Geometry: final body of the model. Coordinates: model frame, mm. A direction names the side the tool comes from. Round coordinates to 2 decimals unless told otherwise and drop trailing zeros. Write each loop counter-clockwise with the first axis right and the second up, starting at its lowest first coordinate (ties: lowest second). Pieces come first, ordered by that corner, then holes. Notation, with made-up numbers: (15.5, 24.25) - (46.5, 24.25) arc R15 ccw to (46.5, 29.25) - close; hole circle Ø6 at (-25.75, 54.25). An arc over 180 degrees is marked (long way). Write each question's results on one line, items separated by ' | '.
from build123d import *

# Parameters (mm, degrees)
SKETCH_2_R               = 15
EXTRUDE_1_DEPTH          = 13
SKETCH_8_R               = 2
CUT_EXTRUDE_10_DEPTH     = 12.5
EXTRUDE_START            = 0.5
SKETCH_10_R              = 15
EXTRUDE_4_DEPTH          = 0.5
SKETCH_11_R              = 12
EXTRUDE_5_DEPTH          = 0.5
SKETCH_12_R              = 5
CUT_EXTRUDE_12_DEPTH     = 26.416530054
FILLET_START             = -0.3000001
FILLET_2_DEPTH           = 13.1000002
FILLET_2_2_ANGLE         = 17.614798
PATTERN_CIRCULAR_1_COUNT = 20


with BuildPart() as part:
    # 草图2 → 凸台-拉伸1 (new body)
    with BuildSketch(Plane(origin=(0, 0, 0), x_dir=(1, 0, 0), z_dir=(0, 1, 0))):
        with Locations(Location((0, 0, 0), (0, 0, 90))):
            Circle(SKETCH_2_R)
    extrude(amount=EXTRUDE_1_DEPTH)

    # 草图8 → 切除-拉伸10 (cut)
    with BuildSketch(Plane.XZ):
        with Locations((0, 15)):
            Circle(SKETCH_8_R)
    cut_extrude_10 = extrude(amount=-CUT_EXTRUDE_10_DEPTH, mode=Mode.SUBTRACT)

    # 草图10 → 凸台-拉伸4 (add)
    with BuildSketch(Plane.XZ.offset(EXTRUDE_START)):
        with Locations(Location((0, 0, 0), (0, 0, 270))):
            Circle(SKETCH_10_R)
    extrude(amount=-EXTRUDE_4_DEPTH)

    # 草图11 → 凸台-拉伸5 (add)
    with BuildSketch(Plane.XZ.offset(0.5)):
        with Locations(Location((0, 0, 0), (0, 0, 270))):
            Circle(SKETCH_11_R)
    extrude(amount=EXTRUDE_5_DEPTH)

    # 草图12 → 切除-拉伸12 (cut, through all)
    with BuildSketch(Plane.XZ.offset(1)):
        with Locations(Location((0, 0, 0), (0, 0, 270))):
            Circle(SKETCH_12_R)
    extrude(amount=-CUT_EXTRUDE_12_DEPTH, mode=Mode.SUBTRACT)

    # 圆角2: read off the stored shape, not the designer's step
    # 圆角2 outline → 圆角2 (cut)
    with BuildSketch(Plane(origin=(0, 0, 0), x_dir=(1, 0, 0), z_dir=(0, 1, 0)).offset(FILLET_START)):
        with BuildLine():
            ThreePointArc((2.296701806, -14.823129252), (2.080163818, -14.773434354), (1.957189365, -14.588405797))
            ThreePointArc((1.957189365, -14.588405797), (0, -13), (-1.957189365, -14.588405797))
            ThreePointArc((-1.957189365, -14.588405797), (-2.080163818, -14.773434354), (-2.296701806, -14.823129252))
            ThreePointArc((-2.296701806, -14.823129252), (0, -15), (2.296701806, -14.823129252))
        make_face()
    extrude(amount=FILLET_2_DEPTH, mode=Mode.SUBTRACT)

    # Fillet 2 2 outline → Fillet 2 2 (revolve)
    with BuildSketch(Plane(origin=(0, 0, 0), x_dir=(-0.1531134537578896, 0, 0.9882086167800453), z_dir=(-0.9882086167800453, 0, -0.1531134537578896))):
        with BuildLine():
            Line((13, 12.8000001), (13, 12.5))
            Line((13, 12.5), (14.7, 12.5))
            ThreePointArc((14.7, 12.5), (14.912132034, 12.587867966), (15, 12.8))
            Line((15, 12.8), (13, 12.8000001))
        make_face()
        with BuildLine():
            Line((14.7, 0), (13, 0))
            Line((13, 0), (13, -0.3000001))
            Line((13, -0.3000001), (15, -0.3))
            ThreePointArc((15, -0.3), (14.912132034, -0.087867966), (14.7, 0))
        make_face()
    revolve(axis=Axis((0, 0, 0), (0, 1, 0)), revolution_arc=FILLET_2_2_ANGLE)

    # 阵列(圆周)1: 切除-拉伸10 ×20 about axis
    pattern_circular_1_axis = Axis((0, 0, 0), (0, 1, 0))
    for i in range(1, PATTERN_CIRCULAR_1_COUNT):
        add(cut_extrude_10.rotate(pattern_circular_1_axis, i * 360 / PATTERN_CIRCULAR_1_COUNT), mode=Mode.SUBTRACT)


solid = part.part
Q1. Section query C-C, the plane x = 9.25. Return loops of the section in (y, z), plus the area to 3 significant figures.
Answer block:
outline: (-1, -7.64) - (-0.5, -7.64) - (-0.5, -11.81) - (0, -11.81) - (0, -10.18) - (12.5, -10.18) - (12.5, -11.81) - (13, -11.81) - (13, 11.81) - (12.5, 11.81) - (12.5, 10.18) - (0, 10.18) - (0, 11.81) - (-0.5, 11.81) - (-0.5, 7.64) - (-1, 7.64) - close | area: 286 mm2
Q2. Ray query, line 1 along Y through (x, z) = (1, 13.5); line 2 along X through (y, z) = (6.75, 0); line 3 along X through (y, z) = (3.5, 10.5). Return the intervals inside material, ascending.
Answer block:
line 1: -0.5 to 0, 12.5 to 13 | line 2: -13 to -5, 5 to 13 | line 3: -10.71 to -9.97, -7.67 to 7.67, 9.97 to 10.71
Q3. Pin query (flat end, axial travel): pin 1 (1.5 mm diameter, centred on x = -11, z = 9, fed in from -Y); pin 2 (3 mm diameter, centred on x = -11.5, y = 8, fed in from -Z); pin 3 (8 mm diameter, centred on x = -5.5, y = 9, fed in from -Z). Return the tip coordinate at first contact, or that it passes through.
Answer block:
pin 1: y = -0.5 | pin 2: z = -10.85 | pin 3: z = -14.87
Q4. Access query for faces 4 (the cylindrical face through (7.68, 6.16, -10.49)), 5 (the flat face through (14, 0, 0)), 6 (the flat face through (-14, 12.5, 0)), 7 (the flat face through (0, 0, -14)). Directions: +Z, -Z, +X, -X, +Y, -Y. A direction counts if a zero-diameter tool reaches every point of the face in a straight line with its end or side. Return the directions, or none.
Answer block:
face 4: none | face 5: +X | face 6: -X | face 7: -Z
Q5. Mould query, pull axis Z, two halves, no side actions, for faces 1 (the cylindrical face through (0, 6, 13)), 2 (the cylindrical face through (3.977, 6.162, 12.377)), 3 (the flat face through (10, -0.5, 7)). Classes: pulls with the +Z half, pulls with the -Z half, needs draft (parallel to the pull), parting line crosses it, or undercut.
Answer block:
face 1: pulls with the +Z half | face 2: undercut | face 3: needs draft
Q6. Section query A-A, the plane z = 0. Return loops of the section in (x, y).
Answer block:
outline: (-15, -0.5) - (-12, -0.5) - (-12, -1) - (-5, -1) - (-5, 13) - (-15, 13) - (-15, 12.5) - (-13, 12.5) - (-13, 0) - (-15, 0) - close; (5, -1) - (12, -1) - (12, -0.5) - (15, -0.5) - (15, 0) - (13, 0) - (13, 12.5) - (15, 12.5) - (15, 13) - (5, 13) - close
Q7. Section query D-D, the plane z = 3.5. Return loops of the section in (x, y), plus the area to 3 significant figures.
Answer block:
outline: (-14.59, -0.5) - (-11.48, -0.5) - (-11.48, -1) - (-3.57, -1) - (-3.57, 13) - (-14.59, 13) - (-14.59, 12.5) - (-12.62, 12.5) - (-12.62, 0) - (-14.59, 0) - close; (3.57, -1) - (11.48, -1) - (11.48, -0.5) - (14.59, -0.5) - (14.59, 0) - (12.62, 0) - (12.62, 12.5) - (14.59, 12.5) - (14.59, 13) - (3.57, 13) - close | area: 256 mm2
Q8. Section query B-B, the plane x = 0. Return loops of the section in (y, z), plus the area to 3 significant figures.
Answer block:
outline: (-1, -12) - (-0.5, -12) - (-0.5, -15) - (0, -15) - (0, -13) - (12.5, -13) - (12.5, -15) - (13, -15) - (13, -5) - (-1, -5) - close; (-1, 5) - (13, 5) - (13, 15) - (12.8, 15) arc R0.3 ccw to (12.5, 14.7) - (12.5, 13) - (0, 13) - (0, 14.7) arc R0.3 ccw to (-0.3, 15) - (-0.5, 15) - (-0.5, 12) - (-1, 12) - close | area: 227 mm2
